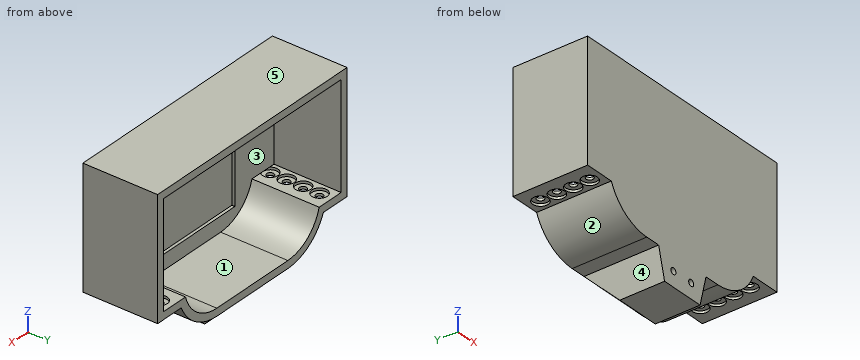
from build123d import *

# Parameters (mm, degrees)
BOSS_EXTRUDE1_DEPTH     = 50
SHELL1_T                = -5
SKETCH2_W               = 84
SKETCH2_H               = 65
CUT_EXTRUDE1_DEPTH      = 2
BOSS_EXTRUDE2_DEPTH     = 45
CHAMFER1_SIZE           = 20
HOLE1_D                 = 4.25
HOLE1_CBORE_D           = 10.25
HOLE1_CBORE_DEPTH       = 40
SKETCH9_R               = 5.159375
CUT_EXTRUDE2_DEPTH      = 1.6491
SKETCH11_R              = 2.38125
CUT_EXTRUDE3_DEPTH      = 5
MIRROR2_COPY_1_SKETCH_R = 5.159375
MIRROR2_COPY_1_DEPTH    = 1.6491


with BuildPart() as part:
    # Sketch1 → Boss-Extrude1 (new body)
    with BuildSketch(Plane(origin=(0, 0, 0), x_dir=(1, 0, 0), z_dir=(0, 1, 0))):
        with BuildLine():
            Line((0, 0), (160, 0))
            Line((160, 0), (160, 80))
            Line((160, 80), (140, 80))
            ThreePointArc((140, 80), (128.027756377, 94.541634566), (110, 100))
            Line((110, 100), (100, 100))
            Line((100, 100), (95, 120))
            Line((95, 120), (65, 120))
            Line((65, 120), (60, 100))
            Line((60, 100), (50, 100))
            ThreePointArc((50, 100), (31.972243623, 94.541634566), (20, 80))
            Line((20, 80), (0, 80))
            Line((0, 80), (0, 0))
        make_face()
    extrude(amount=BOSS_EXTRUDE1_DEPTH)

    # Shell1
    shell1_openings = [part.faces().sort_by_distance(p)[0] for p in [
        (80, 50, -49.668654168),
    ]]
    offset(amount=SHELL1_T, openings=shell1_openings, kind=Kind.INTERSECTION)

    # Sketch2 → Cut-Extrude1 (cut)
    with BuildSketch(Plane(origin=(0, 5, 0), x_dir=(1, 0, 0), z_dir=(0, 1, 0))):
        with Locations((80, 52.5)):
            Rectangle(SKETCH2_W, SKETCH2_H)
    extrude(amount=-CUT_EXTRUDE1_DEPTH, mode=Mode.SUBTRACT)

    # Sketch3 → Boss-Extrude2 (add)
    with BuildSketch(Plane(origin=(0, 5, 0), x_dir=(1, 0, 0), z_dir=(0, 1, 0))):
        Polygon((65, 120), (60, 100), (60, 95), (100, 95), (100, 100), (95, 120), align=None)
    extrude(amount=BOSS_EXTRUDE2_DEPTH)

    # Chamfer1
    chamfer1_edges = [part.edges().sort_by_distance(p)[0] for p in [
        (80, 50, -120),
    ]]
    chamfer(chamfer1_edges, length=CHAMFER1_SIZE)

    # Hole1 (through all)
    with Locations(Plane(origin=(72.5, 50, -110), x_dir=(0, 0, 1), z_dir=(0, 1, 0))):
        with Locations((0, 0), (0, 15)):
            CounterBoreHole(HOLE1_D / 2, HOLE1_CBORE_D / 2, HOLE1_CBORE_DEPTH)

    # Sketch9 → Cut-Extrude2 (cut)
    with BuildSketch(Plane(origin=(0, 0, -80), x_dir=(-1, 0, 0), z_dir=(0, 0, -1))):
        with Locations((-147.5, 41.5)):
            Circle(SKETCH9_R)
        with Locations((-147.5, 30.5)):
            Circle(SKETCH9_R)
        with Locations((-147.5, 19.5)):
            Circle(SKETCH9_R)
        with Locations((-147.5, 8.5)):
            Circle(SKETCH9_R)
    cut_extrude2 = extrude(amount=-CUT_EXTRUDE2_DEPTH, mode=Mode.SUBTRACT)

    # Mirror1: Cut-Extrude2 across plane
    add(cut_extrude2.mirror(Plane.XY.offset(-77.5)), mode=Mode.SUBTRACT)

    # Sketch11 → Cut-Extrude3 (cut)
    with BuildSketch(Plane(origin=(0, 0, -80), x_dir=(-1, 0, 0), z_dir=(0, 0, -1))):
        with Locations((-147.5, 41.5)):
            Circle(SKETCH11_R)
        with Locations((-147.5, 30.5)):
            Circle(SKETCH11_R)
        with Locations((-147.5, 19.5)):
            Circle(SKETCH11_R)
        with Locations((-147.5, 8.5)):
            Circle(SKETCH11_R)
    cut_extrude3 = extrude(amount=-CUT_EXTRUDE3_DEPTH, mode=Mode.SUBTRACT)

    # Mirror2: Cut-Extrude2, Cut-Extrude3 across plane
    add(cut_extrude2.mirror(Plane(origin=(80, 0, 0), x_dir=(0, 0, 1), z_dir=(1, 0, 0))), mode=Mode.SUBTRACT)
    add(cut_extrude3.mirror(Plane(origin=(80, 0, 0), x_dir=(0, 0, 1), z_dir=(1, 0, 0))), mode=Mode.SUBTRACT)

    # Mirror2 copy 1 sketch → Mirror2 copy 1 (cut)
    with BuildSketch(Plane(origin=(160, 0, -75), x_dir=(1, 0, 0), z_dir=(0, 0, 1))):
        with Locations((-147.5, 41.5)):
            Circle(MIRROR2_COPY_1_SKETCH_R)
        with Locations((-147.5, 30.5)):
            Circle(MIRROR2_COPY_1_SKETCH_R)
        with Locations((-147.5, 19.5)):
            Circle(MIRROR2_COPY_1_SKETCH_R)
        with Locations((-147.5, 8.5)):
            Circle(MIRROR2_COPY_1_SKETCH_R)
    extrude(amount=-MIRROR2_COPY_1_DEPTH, mode=Mode.SUBTRACT)


solid = part.part
Input: part model. Units: mm. Frame: model coordinates. Face numbers are marked on the shaded views. A direction names the side the tool comes from. Round coordinates to 2 decimals unless told otherwise and drop trailing zeros. Order: outer loops, then holes, each group sorted by start corner. A loop starts at its lowest first (then second) coordinate and runs counter-clockwise, first axis right, second up.
1. Pin query (flat end, axial travel): P1, Ø11.5, axis at x = 146.5, y = 28, coming from the -Z side; P2, Ø11.5, axis at x = 88.5, z = -110.5, coming from the +Y side; P3, Ø6, axis at x = 27, y = 26, coming from the -Z side. Return the tip coordinate at first contact, or that it passes through.
The answers:
P1: stops at z = -80
P2: stops at y = 45.25
P3: stops at z = -93.12
2. Cut plane B-B, the plane x = 72.5. Output: boundary loops of the cut face in (y, z) (3 decimals), then the cut area to 3 significant figures.
The answers:
outline: (0, -120) - (30, -120) - (34.875, -115.125) - (10, -115.125) - (10, -112.125) - (0, -112.125) - close; (0, -107.875) - (10, -107.875) - (10, -104.875) - (45.125, -104.875) - (50, -100) - (50, -95) - (5, -95) - (5, -85) - (3, -85) - (3, -20) - (5, -20) - (5, -5) - (50, -5) - (50, 0) - (0, 0) - close
area: 1,270 mm2
3. Cut plane C-C, the plane x = 124.5. Output: boundary loops of the cut face in (y, z).
The answers:
outline: (0, -96.59) - (50, -96.59) - (50, -90.87) - (5, -90.87) - (5, -5) - (50, -5) - (50, 0) - (0, 0) - close
4. Cut plane D-D, the plane x = 26.5. Output: boundary loops of the cut face in (y, z), then the cut area to 3 significant figures.
The answers:
outline: (0, -89.95) - (50, -89.95) - (50, -81.78) - (5, -81.78) - (5, -5) - (50, -5) - (50, 0) - (0, 0) - close
area: 1,040 mm2
5. Mould query, pull axis X, two halves, no side actions, for the marked faces 3, 4 and 5. Classes: released by +X, released by -X, zero draft, split by the parting line, or undercut.
The answers:
face 3: undercut
face 4: released by -X
face 5: zero draft
6. Material intervals for line 1 (Y direction, x = 12.5, z = -77); line 2 (Y direction, x = 147.5, z = -79.5); line 3 (X direction, y = 16, z = -71), sorted ascending.
The answers:
line 1: y = 0 to 6.12, 10.88 to 17.12, 21.88 to 28.12, 32.88 to 39.12, 43.88 to 50
line 2: y = 0 to 3.34, 13.66 to 14.34, 24.66 to 25.34, 35.66 to 36.34, 46.66 to 50
line 3: x = 0 to 5, 155 to 160
7. Cut plane A-A, the plane x = 147.5. State how many separate pieces and enclosed holes the cut face has, then the cut area to 3 significant figures.
The answers:
separate pieces: 5
enclosed holes: 0
area: 681 mm2
8. Set-up query: the marked faces 1 and 2. Return all of +Z, -Z, +X, -X, +Y, -Y with unobstructed straight access to the full face (end or side cutting, diameter ignored); none if empty.
The answers:
face 1: +Y
face 2: -Z, -X, +Y, -Y
